Could you check a few things on this drawing? It's one solid part, dimensions in mm from its lowest x, y, z. A direction names the side the tool comes from. Give positions to 0.01 mm unless a question says otherwise; leave off trailing zeros. Write each loop counter-clockwise with the first axis right and the second up, starting at its lowest first coordinate (ties: lowest second). Pieces come first, ordered by that corner, then holes. Notation, with made-up numbers: (78, 80.25) -> (109, 80.25) arc R32 ccw to (109, 110.25) -> close; hole circle Ø1 at (-39.5, 86.5). An arc over 180 degrees is marked (long way). Use CSV: the item, a comma, the result in double quotes. Start each with the question number.
(1) Suppose I cut it at C-C on z = 0.4. List the corners of the cut face in (x, y) for me.
(2) Which directions (+Z, -Z, +X, -X, +Y, -Y) give clear straight access to the entire face, cutting with the end or side of a thin tool? Please do the marked faces 1 and 2.
(3) Suppose I cut it at D-D on y = 1.25. List the corners of the cut face in (x, z) for me, plus the area to 3 significant figures.
(4) Suppose I cut it at A-A on y = 2. List the corners of the cut face in (x, z) for me, plus the area to 3 significant figures.
(5) I need wall thicknesses on L1, parallel to X at y = 3.75, z = 1.7; L2, parallel to Y at x = 2.5, z = 2.3; L3, parallel to Y at x = 3.25, z = 3.1. Which ranges of each line are inside material? Lowest first, please. Write a range as [from, to].
(6) If we mould it in two halves opening along Y, with no side actions, what happens to the marked faces 3, 4 and 5? For each: pulls with the +Y half, pulls with the -Y half, needs draft (parallel to the pull), parting line crosses it, or undercut.
(7) Suppose I cut it at B-B on x = 3.25. List the corners of the cut face in (y, z) for me, plus the area to 3 significant figures.
(8) For pin 1 Ø1 at (x, y) = (4, 3) entering from -Z, with a flat end and sliding along its axis, tell me the tip position at first contact or that it passes through.
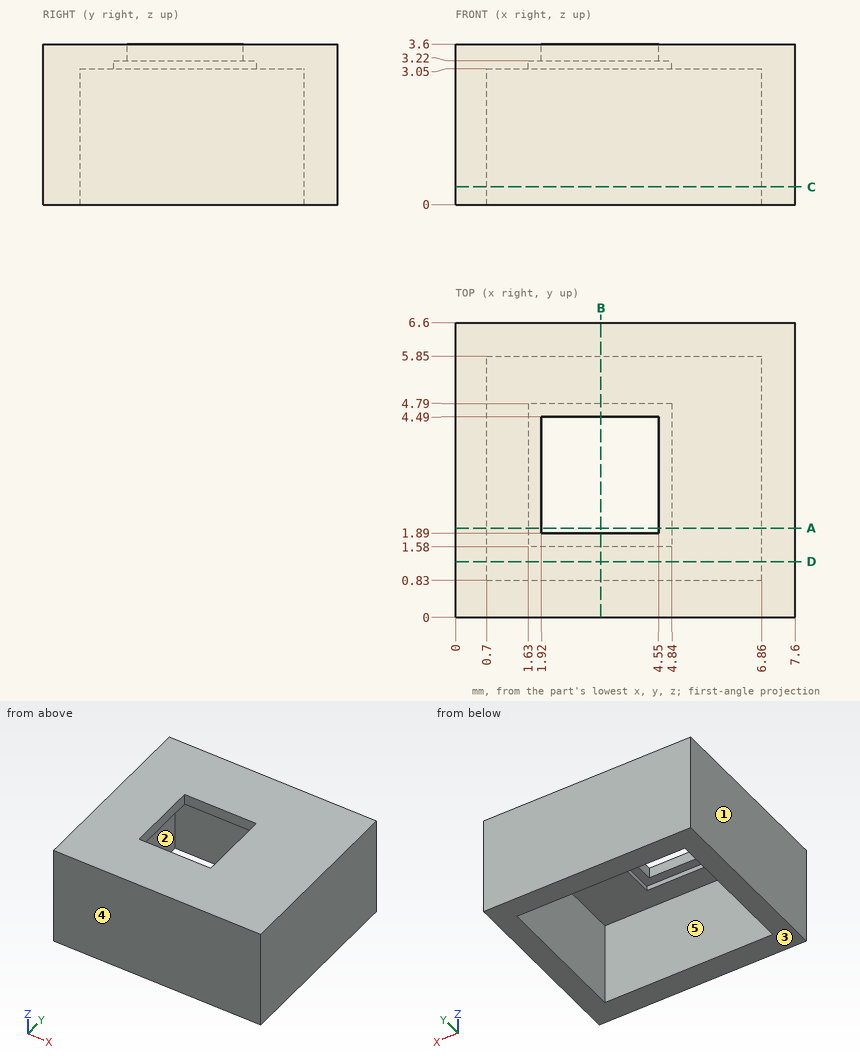
Geometry says:
1,outline,"(0, 0) -> (7.6, 0) -> (7.6, 6.6) -> (0, 6.6) -> close; hole (0.7, 0.83) -> (6.86, 0.83) -> (6.86, 5.85) -> (0.7, 5.85) -> close"
2,face 1,"+Z, -Z, -X, +Y, -Y"
2,face 2,"-Z"
3,outline,"(0, 0) -> (0.7, 0) -> (0.7, 3.05) -> (6.86, 3.05) -> (6.86, 0) -> (7.6, 0) -> (7.6, 3.6) -> (0, 3.6) -> close"
3,area,"8.57 mm²"
4,outline,"(0, 0) -> (0.7, 0) -> (0.7, 3.05) -> (1.63, 3.05) -> (1.63, 3.22) -> (1.92, 3.22) -> (1.92, 3.6) -> (0, 3.6) -> close; (4.55, 3.22) -> (4.84, 3.22) -> (4.84, 3.05) -> (6.86, 3.05) -> (6.86, 0) -> (7.6, 0) -> (7.6, 3.6) -> (4.55, 3.6) -> close"
4,area,"7.03 mm²"
5,L1,"[0, 0.7], [6.86, 7.6]"
5,L2,"[0, 0.83], [5.85, 6.6]"
5,L3,"[0, 1.58], [4.79, 6.6]"
6,face 3,"needs draft"
6,face 4,"pulls with the -Y half"
6,face 5,"undercut"
7,outline,"(0, 0) -> (0.83, 0) -> (0.83, 3.05) -> (1.58, 3.05) -> (1.58, 3.22) -> (1.89, 3.22) -> (1.89, 3.6) -> (0, 3.6) -> close; (4.49, 3.22) -> (4.79, 3.22) -> (4.79, 3.05) -> (5.85, 3.05) -> (5.85, 0) -> (6.6, 0) -> (6.6, 3.6) -> (4.49, 3.6) -> close"
7,area,"6.92 mm²"
8,pin 1,"through"
